```python
from build123d import *

# Parameters (mm, degrees)
SKETCH003_R      = 2.5
EXTRUDE003_DEPTH = 10
EXTRUDE002_DEPTH = 10
EXTRUDE001_DEPTH = 10
SKETCH_R         = 2.5
EXTRUDE_DEPTH    = 10


with BuildPart() as extrude003:
    # Sketch003 (on Cut) → Extrude003 (new body)
    with BuildSketch(Plane.XZ):
        with Locations((9.41, 0)):
            Circle(SKETCH003_R)
        with Locations((29.41, 0)):
            Circle(SKETCH003_R)
    extrude(amount=-EXTRUDE003_DEPTH)


with BuildPart() as extrude002:
    # Sketch002 (on Fusion) → Extrude002 (new body, symmetric)
    with BuildSketch(Plane(origin=(0, 10, 0), x_dir=(1, 0, 0), z_dir=(0, 0, 1))):
        Polygon((15.41, 0), (19.41, -4), (23.41, 0), align=None)
    extrude(amount=EXTRUDE002_DEPTH, both=True)


with BuildPart() as extrude001:
    # Sketch001 (on Extrude) → Extrude001 (new body)
    with BuildSketch(Plane.XZ):
        Polygon((1.91, 0), (36.91, 0), (31.91, -10), (6.91, -10), align=None)
    extrude(amount=-EXTRUDE001_DEPTH)


with BuildPart() as cut001:
    # Sketch → Extrude (new body)
    with BuildSketch(Plane.XY):
        with BuildLine():
            Line((0, 0), (38.81966, 0))
            ThreePointArc((38.81966, 0), (51.90983, 5), (38.81966, 10))
            Line((38.81966, 10), (0, 10))
            ThreePointArc((0, 10), (-13.09017, 5), (0, 0))
        make_face()
        with Locations((-5.59017, 5)):
            Circle(SKETCH_R, mode=Mode.SUBTRACT)
        with Locations((44.40983, 5)):
            Circle(SKETCH_R, mode=Mode.SUBTRACT)
    extrude(amount=EXTRUDE_DEPTH)

    # Fusion: union Extrude001
    add(extrude001.part)

    # Cut: cut Extrude002
    add(extrude002.part, mode=Mode.SUBTRACT)

    # Cut001: cut Extrude003
    add(extrude003.part, mode=Mode.SUBTRACT)


solid = cut001.part
```
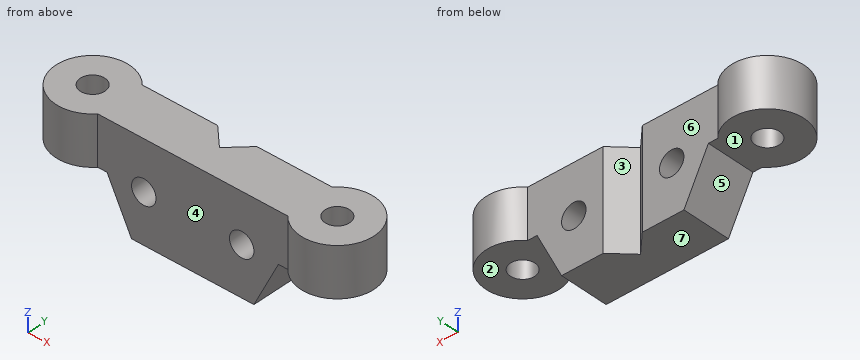
Design review of the part built by this model. Coordinates are the model's own, in mm. Face numbers are marked on the shaded views. A direction names the side the tool comes from. Give positions to 0.01 mm unless a question says otherwise; leave off trailing zeros. Order: outer loops, then holes, each group sorted by start corner. A loop starts at its lowest first (then second) coordinate and runs counter-clockwise, first axis right, second up. Notation, with made-up numbers: M 75.5,-40 L 124.5,-40 A13 ccw 124.5,-28 Z; hole C 36,-23.75 d7. An arc over 180 degrees is marked long. One line per question, with ' | ' between items. Start each with the question number.
Q1. We need section C-C (z = -1.5). Write out the cut boundary in (x, y).
Q2. We need section B-B (y = 5). Write out the cut boundary in (x, z).
Q3. For L1, parallel to Z at x = 9.41, y = 6.75; L2, parallel to Z at x = -8, y = 2, list the stretches that pass through material, from the lowest coordinate up. Write a range as [from, to].
Q4. We need section D-D (z = 8.5). Write out the cut boundary in (x, y).
Q5. The part is to be moulded in two halves that separate along X. For the marked faces 4, 5, 6 and 7, say which applies: +X half, -X half, draft (parallel to the pull), parting line (faces both ways), or undercut.
Q6. We need section A-A (x = 29.41). Write out the cut boundary in (y, z), plus the area to 3 significant figures.
Q7. For pin 1 Ø1.5 at (x, z) = (25, -4.5) entering from -Y; pin 2 Ø5 at (x, z) = (8, -0.5) entering from +Y; pin 3 Ø7.5 at (x, y) = (45.5, 5.5) entering from -Z, all flat-tipped, find the tip position at first contact; note any pin that passes through.
Q8. Machinability: for the marked faces 1, 2 and 3, which of the approach directions +Z, -Z, +X, -X, +Y, -Y give a long, thin tool a straight path to every point of the face, cutting with its end or side? Answer none if there is none.
Returned:
1) outline: M 2.66,0 L 7.41,0 L 7.41,10 L 2.66,10 Z; M 11.41,0 L 27.41,0 L 27.41,10 L 23.41,10 L 19.41,6 L 15.41,10 L 11.41,10 Z; M 31.41,0 L 36.16,0 L 36.16,10 L 31.41,10 Z
2) outline: M -13.09,0 L -8.09,0 L -8.09,10 L -13.09,10 Z; M -3.09,0 L 1.91,0 L 6.91,-10 L 31.91,-10 L 36.91,0 L 41.91,0 L 41.91,10 L -3.09,10 Z; M 46.91,0 L 51.91,0 L 51.91,10 L 46.91,10 Z; hole C 9.41,0 d5; hole C 29.41,0 d5
3) L1: [-10, -2.5], [2.5, 10] | L2: [0, 10]
4) outline: M 0,0 L 38.82,0 A7.5 ccw long 38.82,10 L 23.41,10 L 19.41,6 L 15.41,10 L 0,10 A7.5 ccw long Z; hole C -5.59,5 d5; hole C 44.41,5 d5
5) face 4: undercut | face 5: -X half | face 6: undercut | face 7: draft
6) outline: M 0,-10 L 10,-10 L 10,-2.5 L 0,-2.5 Z; M 0,2.5 L 10,2.5 L 10,10 L 0,10 Z | area: 150 mm2
7) pin 1: y = 0 | pin 2: y = 10 | pin 3: z = 0
8) face 1: -Z, -X, +Y, -Y | face 2: -Z, +X, +Y, -Y | face 3: +Z, -Z, +Y
